Autodesk Inventor part; units mm, degrees
ref_plane "YZ Plane" through (0, 0, 0) normal (1, 0, 0) x (0, 1, 0)
ref_plane "XZ Plane" through (0, 0, 0) normal (0, 1, 0) x (-1, 0, 0)
ref_plane "XY Plane" through (0, 0, 0) normal (0, 0, 1) x (1, 0, 0)
sketch "Sketch3" plane through (0, 0, 0) normal (0, 0, 1) x (1, 0, 0)
  circle A0 centre (0, 0) radius 5
  circle A1 centre (0, 0) radius 6.5
  line L0 (-12.3755, 0) -> (14, 0) construction
  circle A2 centre (12, 0) radius 2.5
  circle A3 centre (-12, 0) radius 2.5
  line L1 (-12.8333, 2.357) -> (-2.1667, 6.1283)
  line L2 (-12.8333, -2.357) -> (-2.1667, -6.1283)
  line L3 (2.1667, 6.1283) -> (12.8333, 2.357)
  line L4 (12.8333, -2.357) -> (2.1667, -6.1283)
  circle A4 centre (-12, 0) radius 1.5
  circle A5 centre (12, 0) radius 1.5
  dimension "d6" = 10
  dimension "d7" = 13
  dimension "d21" = 5
  dimension "d22" = 5
  dimension "d23" = 12
  dimension "d24" = 12
  dimension "d25" = 3
  dimension "d26" = 3
extrude "Extrusion2" add sketch "Sketch3" along normal blind 7 contours A0 | A1
extrude "Extrusion5" add sketch "Sketch3" along normal blind 2 contours A0 | A1 | A1 L3 A2 L4 | A1 L2 A3 L1 | A2 | A3
sketch "Sketch5" plane through (0, 0, 0) normal (0, 0, -1) x (-1, 0, 0)
  point P0 (0, 0)
  point P1 (0.2154, 0.4635)
hole "Hole2" at (-0.2154, 0.4635, 0) direction (0, 0, 1) diameter 10 depth 5 tip angle 118
properties part number "bearingHousing"
Read the model definition and answer for the solid it produces. Units are mm, in the model's axes. A direction names the side the tool comes from. Coordinates: 2 decimals unless noted, no trailing zeros. Loops run counter-clockwise (first coordinate to the right, second up) from the corner with the lowest first, then second, coordinate; pieces in that order, holes last. Notation, with made-up numbers: (44.5, 36) - (72.5, 36) arc R22 cw to (72.5, 61) - close; hole circle Ø3 at (38.5, 25). An arc over 180 degrees is marked (long way). Answer in a Markdown table with one row per item.
Q1. The mould has two halves that part along X. Classify faces 1 (the cylindrical face through (4.666, -0.62, 2.535)), 2 (the flat face through (1.4, -1.4, 7)), 3 (the cylindrical face through (10.5, -0.07, 0.99)), 4 (the flat face through (-7.57, -4.22, 0.99)): pulls with the +X half, pulls with the -X half, needs draft (parallel to the pull), parting line crosses it, or undercut.
Here are the results:
| item | result |
|---|---|
| face 1 | undercut |
| face 2 | needs draft |
| face 3 | undercut |
| face 4 | pulls with the -X half |
Q2. Given P1, Ø2, axis at x = 7.5, z = 2, coming from the +Y side, flat-ended and moving along its own axis, determine where the tip first touches the part or whether it passes through.
Here are the results:
| item | result |
|---|---|
| P1 | stops at y = 4.6 |
Q3. Straight lines are drawn through the part: line 1 along X through (y, z) = (0.75, 6.5); line 2 along Z through (x, y) = (-8, -0.75); line 3 along X through (y, z) = (4.5, 2.75). For each, find the intervals that lie inside material, in ascending order. Write a range as [from, to].
Here are the results:
| item | result |
|---|---|
| line 1 | x = [-6.46, -2.7], [2.27, 6.46] |
| line 2 | z = [0, 2] |
| line 3 | x = [-4.69, -3.17], [2.74, 4.69] |
Q4. Find section B-B on z = 1.25. Write down the section's boundary in (x, y).
Here are the results:
| item | result |
|---|---|
| outline | (-12.83, -2.36) - (-2.17, -6.13) arc R6.5 ccw to (2.17, -6.13) - (12.83, -2.36) arc R2.5 ccw to (12.83, 2.36) - (2.17, 6.13) arc R6.5 ccw to (-2.17, 6.13) - (-12.83, 2.36) arc R2.5 ccw to start; hole circle Ø3 at (-12, 0); hole circle Ø10 at (-0.22, 0.46); hole circle Ø3 at (12, 0) |
Q5. For faces 5 (the cylindrical face through (-6.494, -0.286, 4.229)), 6 (the cylindrical face through (-13.5, -0.07, 0.99)), determine the directions among +Z, -Z, +X, -X, +Y, -Y from which every point of the face is accessible in a straight line to the end or side of a thin tool.
Here are the results:
| item | result |
|---|---|
| face 5 | +Z |
| face 6 | +Z, -Z |
Q6. Find section D-D on y = 0. Count the separate pieces of the cut face and the enclosed holes in it, plus the area to 3 significant figures.
Here are the results:
| item | result |
|---|---|
| separate pieces | 4 |
| enclosed holes | 0 |
| area | 48.0 mm^2 |
Q7. Find section C-C on x = 12. Write down the section's boundary in (y, z).
Here are the results:
| item | result |
|---|---|
| outline | (-2.65, 0) - (-1.5, 0) - (-1.5, 2) - (-2.65, 2) - close; (1.5, 0) - (2.65, 0) - (2.65, 2) - (1.5, 2) - close |
Q8. Find section A-A on x = -11.75. Write down the section's boundary in (y, z).
Here are the results:
| item | result |
|---|---|
| outline | (-2.74, 0) - (-1.48, 0) - (-1.48, 2) - (-2.74, 2) - close; (1.48, 0) - (2.74, 0) - (2.74, 2) - (1.48, 2) - close |
